```python
from build123d import *

# Parameters (mm, degrees)
SKETCH1_R           = 15
BOSS_EXTRUDE1_DEPTH = 80
SKETCH2_R           = 30
BOSS_EXTRUDE2_DEPTH = 5
FILLET1_R           = 5
SKETCH3_R           = 2
CUT_EXTRUDE1_DEPTH  = 5


with BuildPart() as part:
    # Sketch1 → Boss-Extrude1 (new body)
    with BuildSketch(Plane.XY):
        Circle(SKETCH1_R)
    extrude(amount=BOSS_EXTRUDE1_DEPTH)

    # Sketch2 → Boss-Extrude2 (add)
    with BuildSketch(Plane.XY.offset(80)):
        Circle(SKETCH2_R)
    extrude(amount=BOSS_EXTRUDE2_DEPTH)

    # Fillet1
    fillet1_edges = [part.edges().sort_by_distance(p)[0] for p in [
        (-15, 0, 80),
        (-30, 0, 80),
    ]]
    fillet(fillet1_edges, radius=FILLET1_R - 0.0001)  # a hair under: the kernel refuses the full size

    # Sketch3 → Cut-Extrude1 (cut)
    with BuildSketch(Plane(origin=(0, 0, 0), x_dir=(-1, 0, 0), z_dir=(0, 0, -1))):
        with Locations((0, 5)):
            Circle(SKETCH3_R)
        with Locations((0, -5)):
            Circle(SKETCH3_R)
    extrude(amount=-CUT_EXTRUDE1_DEPTH, mode=Mode.SUBTRACT)


solid = part.part
```
Source: CAD feature listing. Evaluate the final solid. Frame: model axes, mm. A direction names the side the tool comes from. Round coordinates to 2 decimals unless told otherwise and drop trailing zeros. Write each loop counter-clockwise with the first axis right and the second up, starting at its lowest first coordinate (ties: lowest second). Pieces come first, ordered by that corner, then holes. Notation, with made-up numbers: M -40,39.5 L 15,39.5 A8 cw 15,45.5 Z; hole C -18.5,-26 d8. An arc over 180 degrees is marked long. Answer as a JSON object with one key per item and string values. Group by question number.
(1) Section query C-C on z = 67. Output: boundary loops of the cut face in (x, y), then the cut area to 3 significant figures.
(2) Mould query, pull axis Y, two halves, no side actions, for faces 3 (the cylindrical face through (-14.985, 0.66, 36.975)), 4 (the flat face through (0, 0, 85)), 5 (the cylindrical face through (0, 7, 2)). Classes: +Y half, -Y half, draft (parallel to the pull), parting line (faces both ways), or undercut.
(3) Reachability of faces 1 (the flat face through (0, 0, 0)), 2 (the flat face through (-11, 17, 80)) from +Z, -Z, +X, -X, +Y, -Y: full face, straight path, thin tool, end or side. Return the list, or none.
(4) Ray query, line 1 (Y direction, x = 0, z = 3.25); line 2 (Z direction, x = -0.5, y = 19.5); line 3 (X direction, y = -0.5, z = 5). Return the intervals inside material, ascending. Write a range as [from, to].
(5) First-contact query: pin 1 (1 mm diameter, centred on y = 6, z = 68.5, fed in from -X); pin 2 (6 mm diameter, centred on x = 7, y = -5.5, fed in from -Z); pin 3 (8 mm diameter, centred on x = 13.5, z = 22, fed in from -Y); pin 4 (1.5 mm diameter, centred on x = -5.5, z = 61.5, fed in from +Y). Flat tips, straight axial feed; report the tip coordinate or a pass-through.
Computed values:
{
 "1": {"outline": "C 0,0 d30", "area": "707 mm^2"},
 "2": {"face 3": "parting line", "face 4": "draft", "face 5": "undercut"},
 "3": {"face 1": "-Z, +X, -X, +Y, -Y", "face 2": "-Z"},
 "4": {"line 1": "[-15, -7], [-3, 3], [7, 15]", "line 2": "[79.98, 85]", "line 3": "[-14.99, 14.99]"},
 "5": {"pin 1": "x = -13.96", "pin 2": "z = 0", "pin 3": "y = -11.61", "pin 4": "y = 14.23"}
}
